from build123d import *

# Parameters (mm, degrees)
F0_W     = 510
F0_H     = 472
F1_DEPTH = 200
F2_W     = 100
F2_H     = 160
F3_DEPTH = 191
F4_W     = 100
F4_H     = 160
F5_DEPTH = 191
F6_W     = 100
F6_H     = 160
F7_DEPTH = 191


with BuildPart() as f1:
    # F0 (on Top) → F1 (new body)
    with BuildSketch(Plane.XY):
        with Locations((-61.286047, -26.417014)):
            Rectangle(F0_W, F0_H)
    extrude(amount=F1_DEPTH)

    # F2 (on face) → F3 (cut)
    with BuildSketch(Plane.XY.offset(200)):
        Polygon((-261.286047, 173.582986), (-286.286047, 173.582986), (-286.286047, -226.417014), (-261.286047, -226.417014), (-261.286047, -216.417014), (-161.286047, -216.417014), (-161.286047, -226.417014), (-136.286047, -226.417014), (-136.286047, 173.582986), (-161.286047, 173.582986), (-161.286047, 163.582986), (-261.286047, 163.582986), align=None)
        with Locations((-210.600971, -121.426403)):
            Rectangle(F2_W, F2_H, mode=Mode.SUBTRACT)
        with Locations((-210.732838, 58.589107)):
            Rectangle(F2_W, F2_H, mode=Mode.SUBTRACT)
    extrude(amount=-F3_DEPTH, mode=Mode.SUBTRACT)

    # F4 (on face) → F5 (cut)
    with BuildSketch(Plane.XY.offset(200)):
        Polygon((-108.286047, 175.583639), (-133.286047, 175.583639), (-133.286047, -224.416361), (-108.286047, -224.416361), (-108.286047, -214.416361), (-8.286047, -214.416361), (-8.286047, -224.416361), (16.713953, -224.416361), (16.713953, 175.583639), (-8.286047, 175.583639), (-8.286047, 165.583639), (-108.286047, 165.583639), align=None)
        with Locations((-57.600971, -119.425749)):
            Rectangle(F4_W, F4_H, mode=Mode.SUBTRACT)
        with Locations((-57.732838, 60.589761)):
            Rectangle(F4_W, F4_H, mode=Mode.SUBTRACT)
    extrude(amount=-F5_DEPTH, mode=Mode.SUBTRACT)

    # F6 (on face) → F7 (cut)
    with BuildSketch(Plane.XY.offset(200)):
        Polygon((46.713953, 173.582986), (21.713953, 173.582986), (21.713953, -226.417014), (46.713953, -226.417014), (46.713953, -216.417014), (146.713953, -216.417014), (146.713953, -226.417014), (171.713953, -226.417014), (171.713953, 173.582986), (146.713953, 173.582986), (146.713953, 163.582986), (46.713953, 163.582986), align=None)
        with Locations((97.399029, -121.426403)):
            Rectangle(F6_W, F6_H, mode=Mode.SUBTRACT)
        with Locations((97.267162, 58.589107)):
            Rectangle(F6_W, F6_H, mode=Mode.SUBTRACT)
    extrude(amount=-F7_DEPTH, mode=Mode.SUBTRACT)


solid = f1.part
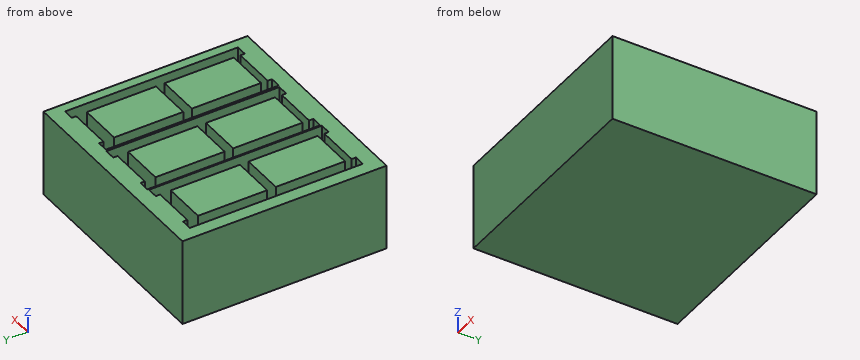
Geometry check sheet. Reference: the model listing, model coordinates, mm. Round coordinates to 2 decimals unless told otherwise and drop trailing zeros. Order: outer loops, then holes, each group sorted by start corner. A loop starts at its lowest first (then second) coordinate and runs counter-clockwise, first axis right, second up. Notation, with made-up numbers: (38.25, -38) - (51.25, -38) arc R24 cw to (51.25, -3) - close; hole circle Ø3 at (30, -25.75). An arc over 180 degrees is marked (long way). One line per question, with ' | ' between items. Start each with the question number.
(1) Sectioned sample at C-C on y = -95. Record the cut outline in (x, z).
(2) Sectioned sample at B-B on x = -47.5. Record the cut outline in (y, z).
(3) Sectioned sample at A-A on z = 124. Count the separate pieces of the cut face and the enclosed holes in it, and give its area (3 significant figures).
(4) Thickness scan on L1, parallel to Y at x = 78, z = 115; L2, parallel to Y at x = -120.5, z = 149; L3, parallel to X at y = 154, z = 186. Record the ranges inside material, lowest first. Write a range as [from, to].
(5) Sectioned sample at D-D on x = 32.5. Record the cut outline in (y, z).
Conclusion:
1) outline: (-316.29, 0) - (193.71, 0) - (193.71, 200) - (171.71, 200) - (171.71, 9) - (147.4, 9) - (147.4, 200) - (47.4, 200) - (47.4, 9) - (21.71, 9) - (21.71, 200) - (16.71, 200) - (16.71, 9) - (-7.6, 9) - (-7.6, 200) - (-107.6, 200) - (-107.6, 9) - (-133.29, 9) - (-133.29, 200) - (-136.29, 200) - (-136.29, 9) - (-160.6, 9) - (-160.6, 200) - (-260.6, 200) - (-260.6, 9) - (-286.29, 9) - (-286.29, 200) - (-316.29, 200) - close
2) outline: (-262.42, 0) - (209.58, 0) - (209.58, 200) - (165.58, 200) - (165.58, 9) - (140.59, 9) - (140.59, 200) - (-19.41, 200) - (-19.41, 9) - (-39.43, 9) - (-39.43, 200) - (-199.43, 200) - (-199.43, 9) - (-214.42, 9) - (-214.42, 200) - (-262.42, 200) - close
3) separate pieces: 7 | enclosed holes: 3 | area: 163,000 mm2
4) L1: y = [-262.42, -216.42], [-201.43, -41.43], [-21.41, 138.59], [163.58, 209.58] | L2: y = [-262.42, -224.42], [175.58, 209.58] | L3: x = [-316.29, -286.29], [-136.29, -133.29], [16.71, 21.71], [171.71, 193.71]
5) outline: (-262.42, 0) - (209.58, 0) - (209.58, 200) - (173.58, 200) - (173.58, 9) - (-226.42, 9) - (-226.42, 200) - (-262.42, 200) - close
